from build123d import *

# Parameters (mm, degrees)
SKETCH_1_W                     = 600
SKETCH_1_H                     = 576
EXTRUDE_1_DEPTH                = 30
SKETCH_2_W                     = 70
SKETCH_2_H                     = 370
CUT_EXTRUDE_1_DEPTH            = 10
SKETCH_3_W                     = 50
SKETCH_3_H                     = 350
CUT_EXTRUDE_2_DEPTH            = 417.346009948
HOLE_WIZARD_M6_1_D             = 6
HOLE_WIZARD_M6_1_DEPTH         = 17
HOLE_WIZARD_M6_1_TIP           = 1.802581857
HOLE_WIZARD_M6_2_AT_2_COUNT    = 2
HOLE_WIZARD_M6_2_AT_2_PITCH    = 147.5
HOLE_WIZARD_M6_2_AT_3_COUNT    = 2
HOLE_WIZARD_M6_2_AT_3_PITCH    = 295
HOLE_WIZARD_M6_3_AT_2_COUNT    = 2
HOLE_WIZARD_M6_3_AT_2_PITCH    = 80
HOLE_WIZARD_M6_3_AT_3_COUNT    = 2
HOLE_WIZARD_M6_3_AT_3_PITCH    = 240
HOLE_WIZARD_M6_3_AT_4_COUNT    = 2
HOLE_WIZARD_M6_3_AT_4_PITCH    = 320
HOLE_WIZARD_M6_1_2_D           = 6.6
HOLE_WIZARD_M6_1_2_CBORE_D     = 13
HOLE_WIZARD_M6_1_2_CBORE_DEPTH = 0.5


with BuildPart() as part:
    # 草图1 → 凸台-拉伸1 (new body)
    with BuildSketch(Plane(origin=(0, 0, 0), x_dir=(1, 0, 0), z_dir=(0, 1, 0))):
        Rectangle(SKETCH_1_W, SKETCH_1_H)
    extrude(amount=EXTRUDE_1_DEPTH)

    # 草图2 → 切除-拉伸1 (cut)
    with BuildSketch(Plane.XZ):
        with BuildLine():
            Line((-245, 75), (-245, -75))
            ThreePointArc((-245, -75), (-150, -170), (-55, -75))
            Line((-55, -75), (-55, 75))
            ThreePointArc((-55, 75), (-150, 170), (-245, 75))
        make_face()
        with Locations((200, 0)):
            Rectangle(SKETCH_2_W, SKETCH_2_H)
        with BuildLine():
            Line((-45, 75), (-45, -75))
            ThreePointArc((-45, -75), (50, -170), (145, -75))
            Line((145, -75), (145, 75))
            ThreePointArc((145, 75), (50, 170), (-45, 75))
        make_face()
    extrude(amount=-CUT_EXTRUDE_1_DEPTH, mode=Mode.SUBTRACT)

    # 草图3 → 切除-拉伸2 (cut, through all)
    with BuildSketch(Plane.XZ.offset(-10)):
        with BuildLine():
            Line((-35, 75), (-35, -75))
            ThreePointArc((-35, -75), (50, -160), (135, -75))
            Line((135, -75), (135, 75))
            ThreePointArc((135, 75), (50, 160), (-35, 75))
        make_face()
        with BuildLine():
            Line((-65, 75), (-65, -75))
            ThreePointArc((-65, -75), (-150, -160), (-235, -75))
            Line((-235, -75), (-235, 75))
            ThreePointArc((-235, 75), (-150, 160), (-65, 75))
        make_face()
        with Locations((200, 0)):
            Rectangle(SKETCH_3_W, SKETCH_3_H)
    extrude(amount=-CUT_EXTRUDE_2_DEPTH, mode=Mode.SUBTRACT)

    # Hole Wizard M6 _1
    with Locations(Plane(origin=(0, 0, 0), x_dir=(-1, 0, 0), z_dir=(0, -1, 0))):
        with Locations((294, -264.5), (294, -223.5), (-294, -264.5), (-294, -223.5), (-294, 264.5), (-294, 223.5), (294, 223.5), (294, 264.5)):
            Hole(HOLE_WIZARD_M6_1_D / 2, depth=HOLE_WIZARD_M6_1_DEPTH)
            with Locations((0, 0, -(HOLE_WIZARD_M6_1_DEPTH + HOLE_WIZARD_M6_1_TIP / 2))):  # 118° drill point
                Cone(0, HOLE_WIZARD_M6_1_D / 2, HOLE_WIZARD_M6_1_TIP, mode=Mode.SUBTRACT)

    # 草图19 → M6 螺纹孔2 (revolve, cut)
    with BuildSketch(Plane(origin=(147.5, 15, -288), x_dir=(0, 1, 0), z_dir=(1, 0, 0))):
        Polygon((0, 0), (0, 11.502151548), (2.5, 10), (2.5, 0), align=None)
    hole_wizard_m6_2 = revolve(axis=Axis((147.5, 15, -294.35), (0, 0, 1)), mode=Mode.SUBTRACT)

    # M6 螺纹孔2 at 2: M6 螺纹孔2 ×2
    with Locations(*[(-i * HOLE_WIZARD_M6_2_AT_2_PITCH, 0, 0) for i in range(1, HOLE_WIZARD_M6_2_AT_2_COUNT)]):
        add(hole_wizard_m6_2, mode=Mode.SUBTRACT)

    # M6 螺纹孔2 at 3: M6 螺纹孔2 ×2
    with Locations(*[(-i * HOLE_WIZARD_M6_2_AT_3_PITCH, 0, 0) for i in range(1, HOLE_WIZARD_M6_2_AT_3_COUNT)]):
        add(hole_wizard_m6_2, mode=Mode.SUBTRACT)

    # 镜向1: M6 螺纹孔2 across plane
    add(hole_wizard_m6_2.mirror(Plane.XY), mode=Mode.SUBTRACT)

    # 镜向1 copy 1 sketch → 镜向1 copy 1 (revolve, cut)
    with BuildSketch(Plane(origin=(0, 15, 288), x_dir=(0, 1, 0), z_dir=(1, 0, 0))):
        Polygon((0, 0), (0, -11.502151548), (2.5, -10), (2.5, 0), align=None)
    revolve(axis=Axis((0, 15, 294.35), (0, 0, 1)), mode=Mode.SUBTRACT)

    # 镜向1 copy 2 sketch → 镜向1 copy 2 (revolve, cut)
    with BuildSketch(Plane(origin=(-147.5, 15, 288), x_dir=(0, 1, 0), z_dir=(1, 0, 0))):
        Polygon((0, 0), (0, -11.502151548), (2.5, -10), (2.5, 0), align=None)
    revolve(axis=Axis((-147.5, 15, 294.35), (0, 0, 1)), mode=Mode.SUBTRACT)

    # 草图22 → M6 螺纹孔3 (revolve, cut)
    with BuildSketch(Plane(origin=(-300, 15, -158), x_dir=(0, 0, 1), z_dir=(0, 1, 0))):
        Polygon((0, 0), (0, 16.502151548), (2.5, 15), (2.5, 0), align=None)
    hole_wizard_m6_3 = revolve(axis=Axis((-306.35, 15, -158), (1, 0, 0)), mode=Mode.SUBTRACT)

    # M6 螺纹孔3 at 2: M6 螺纹孔3 ×2
    with Locations(*[(0, 0, i * HOLE_WIZARD_M6_3_AT_2_PITCH) for i in range(1, HOLE_WIZARD_M6_3_AT_2_COUNT)]):
        add(hole_wizard_m6_3, mode=Mode.SUBTRACT)

    # M6 螺纹孔3 at 3: M6 螺纹孔3 ×2
    with Locations(*[(0, 0, i * HOLE_WIZARD_M6_3_AT_3_PITCH) for i in range(1, HOLE_WIZARD_M6_3_AT_3_COUNT)]):
        add(hole_wizard_m6_3, mode=Mode.SUBTRACT)

    # M6 螺纹孔3 at 4: M6 螺纹孔3 ×2
    with Locations(*[(0, 0, i * HOLE_WIZARD_M6_3_AT_4_PITCH) for i in range(1, HOLE_WIZARD_M6_3_AT_4_COUNT)]):
        add(hole_wizard_m6_3, mode=Mode.SUBTRACT)

    # 镜向2: M6 螺纹孔3 across plane
    add(hole_wizard_m6_3.mirror(Plane(origin=(0, 0, 0), x_dir=(0, 0, 1), z_dir=(1, 0, 0))), mode=Mode.SUBTRACT)

    # 镜向2 copy 1 sketch → 镜向2 copy 1 (revolve, cut)
    with BuildSketch(Plane(origin=(300, 15, -78), x_dir=(0, 0, 1), z_dir=(0, 1, 0))):
        Polygon((0, 0), (0, -16.502151548), (2.5, -15), (2.5, 0), align=None)
    revolve(axis=Axis((306.35, 15, -78), (1, 0, 0)), mode=Mode.SUBTRACT)

    # 镜向2 copy 2 sketch → 镜向2 copy 2 (revolve, cut)
    with BuildSketch(Plane(origin=(300, 15, 82), x_dir=(0, 0, 1), z_dir=(0, 1, 0))):
        Polygon((0, 0), (0, -16.502151548), (2.5, -15), (2.5, 0), align=None)
    revolve(axis=Axis((306.35, 15, 82), (1, 0, 0)), mode=Mode.SUBTRACT)

    # 镜向2 copy 3 sketch → 镜向2 copy 3 (revolve, cut)
    with BuildSketch(Plane(origin=(300, 15, 162), x_dir=(0, 0, 1), z_dir=(0, 1, 0))):
        Polygon((0, 0), (0, -16.502151548), (2.5, -15), (2.5, 0), align=None)
    revolve(axis=Axis((306.35, 15, 162), (1, 0, 0)), mode=Mode.SUBTRACT)

    # Hole Wizard M6 _1 2 (through all)
    with Locations(Plane(origin=(0, 30, 0), x_dir=(1, 0, 0), z_dir=(0, 1, 0))):
        with Locations((-285, 183.68), (0, 183.68), (285, 183.68), (-285, -183.68), (0, -183.68), (285, -183.68)):
            CounterBoreHole(HOLE_WIZARD_M6_1_2_D / 2, HOLE_WIZARD_M6_1_2_CBORE_D / 2, HOLE_WIZARD_M6_1_2_CBORE_DEPTH)


solid = part.part
Model file for the job. Use its own axes, mm. A direction names the side the tool comes from. Round coordinates to 2 decimals unless told otherwise and drop trailing zeros. Order: outer loops, then holes, each group sorted by start corner. A loop starts at its lowest first (then second) coordinate and runs counter-clockwise, first axis right, second up.
(1) Band-saw the part on D-D (z = 122). List the corners of the cut face in (x, y), then the cut area to 3 significant figures.
(2) 3-axis set-ups, long thin cutter, end or side, ignore diameter. For faces 4 (the face through (291.2, 29.75, 181.73)), 5 (the face through (174, 10, -13)), 6 (the face through (225, 20, -2)): which of +Z, -Z, +X, -X, +Y, -Y reach the whole face in a straight line?
(3) Drill centre lines: line 1 (X direction, y = 9, z = -59); line 2 (X direction, y = 21.25, z = 183.68); line 3 (Z direction, x = -294, y = 4.75). Where is each one in solid material? Low to high.
(4) Pull direction X, two halves, no side cores. Call faces 1 (the face through (-4, 15, -288)), 2 (the face through (-300, 15, 4)), 3 (the face through (-0.846, 29.754, -190.125)): released by +X, released by -X, zero draft, split by the parting line, or undercut.
(5) Band-saw the part on A-A (z = -41). List the corners of the cut face in (x, y), then the cut area to 3 significant figures.
(6) Band-saw the part on C-C (y = 25). Give the number of separate pieces and of enclosed holes in the cut face, then the cut area to 3 significant figures.
(7) Pin check, flat tips, straight feed: pin 1 (8.5 mm diameter, centred on x = 0, z = 183.68, fed in from +Y); pin 2 (3.5 mm diameter, centred on x = 294, z = 264.5, fed in from -Y). Stop position of each tip, or through.
(8) Band-saw the part on B-B (x = 210). List the corners of the cut face in (y, z).
Verdict:
1. outline: (-300, 0) - (-232.56, 0) - (-232.56, 10) - (-220.82, 10) - (-220.82, 30) - (-300, 30) - close; (-79.18, 10) - (-67.44, 10) - (-67.44, 0) - (-32.56, 0) - (-32.56, 10) - (-20.82, 10) - (-20.82, 30) - (-79.18, 30) - close; (120.82, 10) - (132.56, 10) - (132.56, 0) - (165, 0) - (165, 10) - (175, 10) - (175, 30) - (120.82, 30) - close; (225, 10) - (235, 10) - (235, 0) - (300, 0) - (300, 30) - (225, 30) - close
1. area: 7,330 mm2
2. face 4: +Y
2. face 5: -Y
2. face 6: +Y, -Y
3. line 1: x = -300 to -245, -55 to -45, 145 to 165, 235 to 300
3. line 2: x = -300 to -288.3, -281.7 to -3.3, 3.3 to 281.7, 288.3 to 300
3. line 3: z = -288 to -267.5, -261.5 to -226.5, -220.5 to 220.5, 226.5 to 261.5, 267.5 to 288
4. face 1: zero draft
4. face 2: released by -X
4. face 3: undercut
5. outline: (-300, 0) - (-245, 0) - (-245, 10) - (-235, 10) - (-235, 30) - (-300, 30) - close; (-65, 10) - (-55, 10) - (-55, 0) - (-45, 0) - (-45, 10) - (-35, 10) - (-35, 30) - (-65, 30) - close; (135, 10) - (145, 10) - (145, 0) - (165, 0) - (165, 10) - (175, 10) - (175, 30) - (135, 30) - close; (225, 10) - (235, 10) - (235, 0) - (300, 0) - (300, 30) - (225, 30) - close
5. area: 5,700 mm2
6. separate pieces: 1
6. enclosed holes: 9
6. area: 231,000 mm2
7. pin 1: stops at y = 29.5
7. pin 2: stops at y = 17.75
8. outline: (0, -288) - (30, -288) - (30, -175) - (10, -175) - (10, -185) - (0, -185) - close; (0, 185) - (10, 185) - (10, 175) - (30, 175) - (30, 288) - (0, 288) - close
